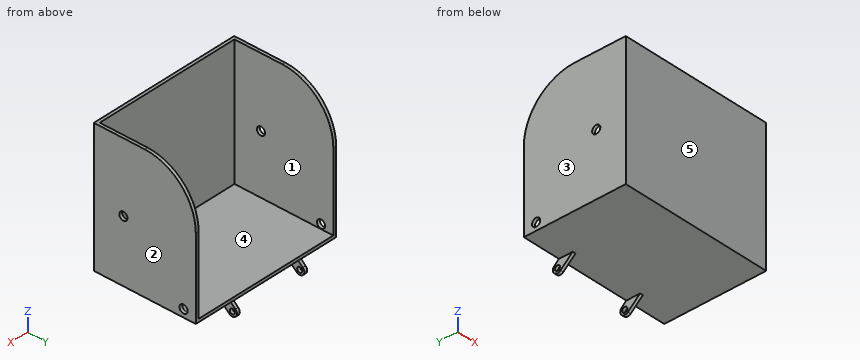
from build123d import *

# Parameters (mm, degrees)
BOSS_EXTRUDE1_DEPTH = 150
SKETCH2_W           = 144
SKETCH2_H           = 132
CUT_EXTRUDE1_DEPTH  = 97
SKETCH3_R           = 2.5
BOSS_EXTRUDE2_DEPTH = 1.5
CUT_EXTRUDE2_REACH  = 227.015
SKETCH4_R           = 4


with BuildPart() as part:
    # Sketch1 → Boss-Extrude1 (new body)
    with BuildSketch(Plane(origin=(0, 0, 0), x_dir=(0, 0, -1), z_dir=(1, 0, 0))):
        with BuildLine():
            Line((0, 0), (-130, 0))
            Line((-130, 0), (-130, 50))
            ThreePointArc((-130, 50), (-115.355339059, 85.355339059), (-80, 100))
            Line((-80, 100), (0, 100))
            Line((0, 100), (0, 0))
        make_face()
    extrude(amount=BOSS_EXTRUDE1_DEPTH)

    # Sketch2 → Cut-Extrude1 (cut)
    with BuildSketch(Plane(origin=(0, 100, 0), x_dir=(1, 0, 0), z_dir=(0, 1, 0))):
        with Locations((75, -69)):
            Rectangle(SKETCH2_W, SKETCH2_H)
    extrude(amount=-CUT_EXTRUDE1_DEPTH, mode=Mode.SUBTRACT)

    # Sketch3 → Boss-Extrude2 (add, symmetric)
    with BuildSketch(Plane(origin=(111, 0, 0), x_dir=(0, 0, -1), z_dir=(1, 0, 0))):
        with BuildLine():
            Line((0, 100), (0, 86.483689179))
            Line((0, 86.483689179), (10.709846007, 98.483689179))
            ThreePointArc((10.709846007, 98.483689179), (10.348889249, 104.837405432), (3.995172996, 104.476448674))
            Line((3.995172996, 104.476448674), (0, 100))
        make_face()
        with Locations((7.352509502, 101.480068927)):
            Circle(SKETCH3_R, mode=Mode.SUBTRACT)
    boss_extrude2 = extrude(amount=BOSS_EXTRUDE2_DEPTH, both=True)

    # Mirror1: Boss-Extrude2 across plane
    add(boss_extrude2.mirror(Plane(origin=(75, 0, 0), x_dir=(0, 0, 1), z_dir=(1, 0, 0))))

    # Sketch4 → Cut-Extrude2 (cut, up to next)
    with BuildSketch(Plane(origin=(150, 0, 0), x_dir=(0, 0, -1), z_dir=(1, 0, 0)), mode=Mode.PRIVATE) as cut_extrude2_sk1:
        with Locations((-61.531516432, 29)):
            Circle(SKETCH4_R)
    cut_extrude2_tool1 = extrude(cut_extrude2_sk1.sketch, amount=-CUT_EXTRUDE2_REACH, mode=Mode.PRIVATE) & part.part
    # Sketch4 → Cut-Extrude2 (cut, up to next)
    with BuildSketch(Plane(origin=(150, 0, 0), x_dir=(0, 0, -1), z_dir=(1, 0, 0)), mode=Mode.PRIVATE) as cut_extrude2_sk2:
        with Locations((-7.503745795, 88)):
            Circle(SKETCH4_R)
    cut_extrude2_tool2 = extrude(cut_extrude2_sk2.sketch, amount=-CUT_EXTRUDE2_REACH, mode=Mode.PRIVATE) & part.part
    cut_extrude2_1 = cut_extrude2_tool1.solids().sort_by_distance((150, 29, 61.531516))[0]
    add(cut_extrude2_1, mode=Mode.SUBTRACT)
    cut_extrude2_2 = cut_extrude2_tool2.solids().sort_by_distance((150, 88, 7.503746))[0]
    add(cut_extrude2_2, mode=Mode.SUBTRACT)
    cut_extrude2 = cut_extrude2_1 + cut_extrude2_2  # Cut-Extrude2 as one shape, for the pattern or mirror that repeats it

    # Mirror2: Cut-Extrude2 across plane
    add(cut_extrude2.mirror(Plane(origin=(75, 0, 0), x_dir=(0, 0, 1), z_dir=(1, 0, 0))), mode=Mode.SUBTRACT)


solid = part.part
Model file for the job. Use its own axes, mm. Face numbers are marked on the shaded views. A direction names the side the tool comes from. Give positions to 0.01 mm unless a question says otherwise; leave off trailing zeros. Order: outer loops, then holes, each group sorted by start corner. A loop starts at its lowest first (then second) coordinate and runs counter-clockwise, first axis right, second up. Notation, with made-up numbers: (-14, 1) - (6, 1) arc R22 ccw to (6, 32) - close; hole circle Ø3 at (-9.75, -34.5). An arc over 180 degrees is marked (long way). Return JSON: item names as keys, results as strings.
1) Cut at A-A, the plane y = 29. Give the cut face in (x, z).
Geometry says:
{"outline": "(0, 0) - (150, 0) - (150, 57.53) - (147, 57.53) - (147, 3) - (3, 3) - (3, 57.53) - (0, 57.53) - close; (0, 65.53) - (3, 65.53) - (3, 130) - (0, 130) - close; (147, 65.53) - (150, 65.53) - (150, 130) - (147, 130) - close"}
2) Cut at B-B, the plane z = 76. Give the cut face in (x, y), plus the area to 3 significant figures.
Geometry says:
{"outline": "(0, 0) - (150, 0) - (150, 100) - (147, 100) - (147, 3) - (3, 3) - (3, 100) - (0, 100) - close", "area": "1,030 mm²"}
3) Probe line 1 (X direction, y = 19.5, z = 13); line 2 (Y direction, x = 35, z = 59). List the from-to ranges inside material, lowest first. Write a range as from..to.
Geometry says:
{"line 1": "0..3, 147..150", "line 2": "0..3"}
4) Cut at C-C, the plane x = 126.5. Give the cut face in (y, z), plus the area to 3 significant figures.
Geometry says:
{"outline": "(0, 0) - (100, 0) - (100, 3) - (3, 3) - (3, 130) - (0, 130) - close", "area": "681 mm²"}
5) 3-axis set-ups, long thin cutter, end or side, ignore diameter. For the marked faces 4 and 5: which of +Z, -Z, +X, -X, +Y, -Y reach the whole face in a straight line?
Geometry says:
{"face 4": "+Z, +Y", "face 5": "+Z, -Z, +X, -X, -Y"}
6) Pull direction X, two halves, no side cores. Call the marked faces 1, 2 and 3: pulls with the +X half, pulls with the -X half, needs draft (parallel to the pull), parting line crosses it, or undercut.
Geometry says:
{"face 1": "undercut", "face 2": "pulls with the +X half", "face 3": "pulls with the -X half"}
7) Cut at D-D, the plane y = 73.5. Give the cut face in (x, z), plus the area to 3 significant figures.
Geometry says:
{"outline": "(0, 0) - (150, 0) - (150, 124.13) - (147, 124.13) - (147, 3) - (3, 3) - (3, 124.13) - (0, 124.13) - close", "area": "1,180 mm²"}
8) Flat gauge pins, fed straight in: P1, Ø12, axis at y = 29, z = 28.5, coming from the -X side; P2, Ø6, axis at y = 95, z = -5, coming from the +X side; P3, Ø8, axis at x = 66.5, y = 22.5, coming from the -Z side; P4, Ø9.5, axis at y = 92, z = -7, coming from the -X side. Where does each tip first touch, or does it go through?
Geometry says:
{"P1": "x = 0", "P2": "x = 112.5", "P3": "z = 0", "P4": "x = 37.5"}
